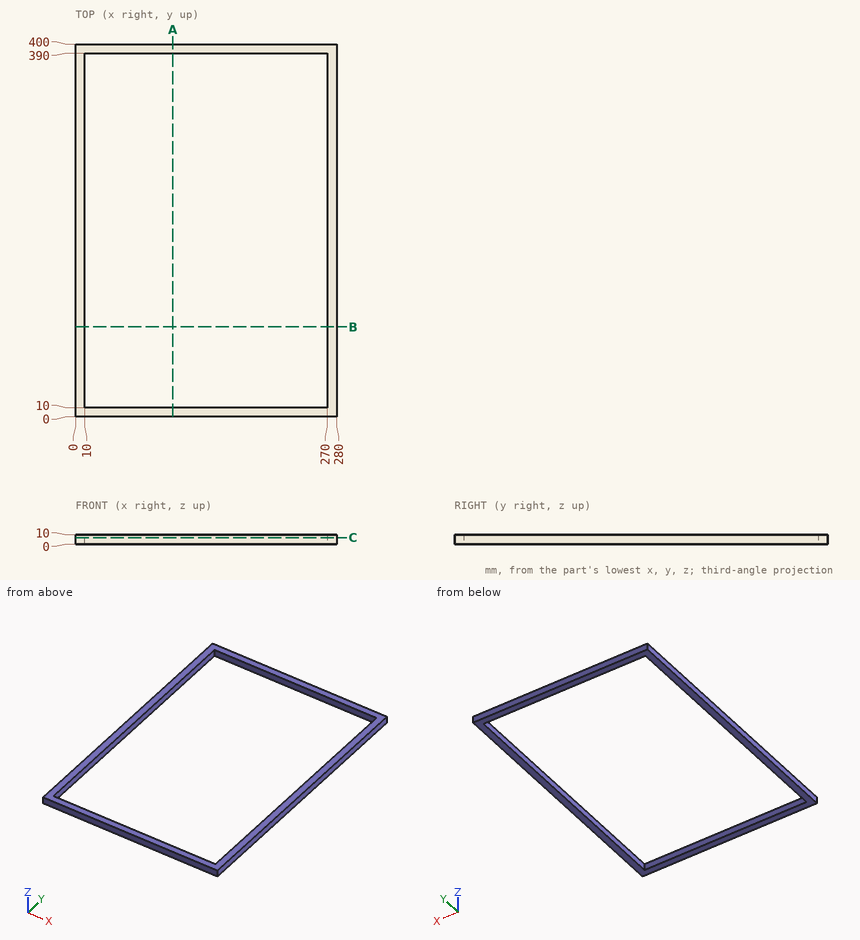
Job drawing, mm, ordinate dimensions from the low corner. One solid piece. Give positions to 0.01 mm unless a question says otherwise; leave off trailing zeros. Write each loop counter-clockwise with the first axis right and the second up, starting at its lowest first coordinate (ties: lowest second). Pieces come first, ordered by that corner, then holes. Notation, with made-up numbers: (71, 26.25) -> (107, 26.25) arc R8 ccw to (107, 41.25) -> close; hole circle Ø9 at (-17.75, 55.25). An arc over 180 degrees is marked (long way). Return JSON: item names as keys, results as strings.
Item 1: Band-saw the part on A-A (x = 104.5). List the corners of the cut face in (y, z), then the cut area to 3 significant figures.
Answer below:
{"outline": "(0, 0) -> (10, 0) -> (10, 10) -> (0, 10) -> close; (390, 0) -> (400, 0) -> (400, 10) -> (390, 10) -> close", "area": "200 mm2"}
Item 2: Band-saw the part on C-C (z = 7.25). List the corners of the cut face in (x, y), then the cut area to 3 significant figures.
Answer below:
{"outline": "(0, 0) -> (280, 0) -> (280, 400) -> (0, 400) -> close; hole (10, 10) -> (270, 10) -> (270, 390) -> (10, 390) -> close", "area": "13,200 mm2"}
Item 3: Drill centre lines: probe 1 along Y at (x, z) = (249, 7); probe 2 along X at (y, z) = (233, 2.5). Where is each one in solid material? Low to high.
Answer below:
{"probe 1": "y = 0 to 10, 390 to 400", "probe 2": "x = 0 to 10, 270 to 280"}
Item 4: Band-saw the part on B-B (y = 96.5). List the corners of the cut face in (x, z), then the cut area to 3 significant figures.
Answer below:
{"outline": "(0, 0) -> (10, 0) -> (10, 10) -> (0, 10) -> close; (270, 0) -> (280, 0) -> (280, 10) -> (270, 10) -> close", "area": "200 mm2"}
